from build123d import *

# Parameters (mm, degrees)
SKETCH1_R           = 3.175
SKETCH1_W           = 25.4
SKETCH1_H           = 50.8
BOSS_EXTRUDE1_DEPTH = 3.175


with BuildPart() as part:
    # Sketch1 → Boss-Extrude1 (new body)
    with BuildSketch(Plane.XY):
        with BuildLine():
            Line((214.219369126, 454.630831078), (392.019369126, 454.630831078))
            ThreePointArc((392.019369126, 454.630831078), (400.999625247, 450.911087199), (404.719369126, 441.930831078))
            Line((404.719369126, 441.930831078), (404.719369126, 340.330831078))
            ThreePointArc((404.719369126, 340.330831078), (400.999625247, 331.350574957), (392.019369126, 327.630831078))
            Line((392.019369126, 327.630831078), (214.219369126, 327.630831078))
            ThreePointArc((214.219369126, 327.630831078), (205.239113005, 331.350574957), (201.519369126, 340.330831078))
            Line((201.519369126, 340.330831078), (201.519369126, 441.930831078))
            ThreePointArc((201.519369126, 441.930831078), (205.239113005, 450.911087199), (214.219369126, 454.630831078))
        make_face()
        with Locations((265.019369126, 406.370831078)):
            Circle(SKETCH1_R, mode=Mode.SUBTRACT)
        with Locations((239.619369126, 431.770831078)):
            Circle(SKETCH1_R, mode=Mode.SUBTRACT)
        with Locations((239.619369126, 380.970831078)):
            Circle(SKETCH1_R, mode=Mode.SUBTRACT)
        with Locations((366.619369126, 380.970831078)):
            Circle(SKETCH1_R, mode=Mode.SUBTRACT)
        with Locations((341.219369126, 406.370831078)):
            Circle(SKETCH1_R, mode=Mode.SUBTRACT)
        with Locations((366.619369126, 431.770831078)):
            Circle(SKETCH1_R, mode=Mode.SUBTRACT)
        with Locations((265.019369126, 355.570831078)):
            Circle(SKETCH1_R, mode=Mode.SUBTRACT)
        with Locations((341.219369126, 355.570831078)):
            Circle(SKETCH1_R, mode=Mode.SUBTRACT)
        with Locations((303.119369126, 406.370831078)):
            Rectangle(SKETCH1_W, SKETCH1_H, mode=Mode.SUBTRACT)
    extrude(amount=BOSS_EXTRUDE1_DEPTH)


solid = part.part
Work out the finished part from the listing and answer in its coordinate system (mm). Give positions to 0.01 mm unless a question says otherwise; leave off trailing zeros. Write each loop counter-clockwise with the first axis right and the second up, starting at its lowest first coordinate (ties: lowest second). Pieces come first, ordered by that corner, then holes.
Q1. Straight lines are drawn through the part: L1, parallel to Y at x = 306, z = 2.9; L2, parallel to X at y = 388.5, z = 2.5; L3, parallel to X at y = 354.5, z = 2.55. For each, find the intervals that lie inside material, in ascending order.
Answer:
L1: y = 327.63 to 380.97, 431.77 to 454.63
L2: x = 201.52 to 290.42, 315.82 to 404.72
L3: x = 201.52 to 262.03, 268.01 to 338.23, 344.21 to 404.72
Q2. The part is cut by section C-C on z = 2.55. State how many separate pieces and enclosed holes the cut face has, and give its area (3 significant figures).
Answer:
separate pieces: 1
enclosed holes: 9
area: 24,100 mm2
Q3. For a pull along Y with two mould halves and no side action, classify faces 1 (the face through (264.33, 352.47, 1.57)), 2 (the face through (205.14, 450.81, 1.57)), 3 (the face through (305, 378, 3.175)) as released by +Y, released by -Y, zero draft, split by the parting line, or undercut.
Answer:
face 1: undercut
face 2: released by +Y
face 3: zero draft
Q4. The part is cut by section B-B on y = 417. Give the vertices of the cut face in (x, z) (3 decimals).
Answer:
outline: (201.519, 0) - (290.419, 0) - (290.419, 3.175) - (201.519, 3.175) - close; (315.819, 0) - (404.719, 0) - (404.719, 3.175) - (315.819, 3.175) - close
Q5. The part is cut by section A-A on x = 298. Give the vertices of the cut face in (y, z) (3 decimals), and give its area (3 significant figures).
Answer:
outline: (327.631, 0) - (380.971, 0) - (380.971, 3.175) - (327.631, 3.175) - close; (431.771, 0) - (454.631, 0) - (454.631, 3.175) - (431.771, 3.175) - close
area: 242 mm2
